from build123d import *

# Parameters (mm, degrees)
F0_W     = 114.3
F0_H     = 127
F0_R     = 38.1
F1_DEPTH = 4.7625
F2_SIZE  = 25.4
F3_SIZE  = 1.524
F4_SIZE  = 3.175


with BuildPart() as f1:
    # F0 (on Top) → F1 (new body, symmetric)
    with BuildSketch(Plane.XY):
        Rectangle(F0_W, F0_H)
        Circle(F0_R, mode=Mode.SUBTRACT)
    extrude(amount=F1_DEPTH, both=True)

    # F2
    f2_edges = [f1.edges().sort_by_distance(p)[0] for p in [
        (57.15, 63.5, 0),
        (-57.15, 63.5, 0),
    ]]
    chamfer(f2_edges, length=F2_SIZE)

    # F3
    f3_edges = [f1.edges().sort_by_distance(p)[0] for p in [
        (-38.1, 0, 4.7625),
        (-38.1, 0, -4.7625),
    ]]
    chamfer(f3_edges, length=F3_SIZE)

    # F4
    f4_edges = [f1.edges().sort_by_distance(p)[0] for p in [
        (0, -63.5, 4.7625),
        (0, -63.5, -4.7625),
    ]]
    chamfer(f4_edges, length=F4_SIZE)


solid = f1.part
Input: part model. Units: mm. Frame: model coordinates. Round coordinates to 2 decimals unless told otherwise and drop trailing zeros. Loops run counter-clockwise (first coordinate to the right, second up) from the corner with the lowest first, then second, coordinate; pieces in that order, holes last. Notation, with made-up numbers: M 82.5,-4 L 138.5,-4 A25 cw 138.5,14 Z; hole C 59.5,30 d10. An arc over 180 degrees is marked long. Answer as CSV lines item,"result". Start each with the question number.
(1) Section B-B, the plane x = 0. Output: boundary loops of the cut face in (y, z) (1 decimal), plus the area to 3 significant figures.
(2) Draft query along Y for faces 1 (the flat face through (-0.8, -61.935, -3.153)), 2 (the flat face through (44.27, 50.98, 0.07)), 3 (the flat face through (-57.15, -13, 0)), 4 (the cylindrical face through (-30.235, -23.183, -0.045)). Return one class per face: released by +Y, released by -Y, zero draft, split by the parting line, or undercut.
(3) Section D-D, the plane y = 43. Output: boundary loops of the cut face in (x, z), plus the area to 3 significant figures.
(4) First-contact query: pin 1 (1 mm diameter, centred on x = 19.5, y = -30, fed in from -Z); pin 2 (2 mm diameter, centred on x = 39.5, z = -3, fed in from -Y); pin 3 (1 mm diameter, centred on x = -37.5, z = 0.5, fed in from +Y). Flat tips, straight axial feed; report the tip coordinate or a pass-through.
(5) Line query: line 1 (Y direction, x = 0, z = 0.5); line 2 (X direction, y = -17.5, z = -0.5); line 3 (Y direction, x = -31, z = -1.25). Output: solid intervals per line, ascending. Write a range as [from, to].
(6) Section A-A, the plane y = 0. Output: boundary loops of the cut face in (x, z), plus the area to 3 significant figures.
Values found:
1,outline,"M -63.5,-1.6 L -60.3,-4.8 L -39.6,-4.8 L -38.1,-3.2 L -38.1,3.2 L -39.6,4.8 L -60.3,4.8 L -63.5,1.6 Z; M 38.1,-3.2 L 39.6,-4.8 L 63.5,-4.8 L 63.5,4.8 L 39.6,4.8 L 38.1,3.2 Z"
1,area,"469 mm²"
2,face 1,"released by -Y"
2,face 2,"released by +Y"
2,face 3,"zero draft"
2,face 4,"undercut"
3,outline,"M -52.25,-4.76 L 52.25,-4.76 L 52.25,4.76 L -52.25,4.76 Z"
3,area,"995 mm²"
4,pin 1,"passes through"
4,pin 2,"stops at y = -63.09"
4,pin 3,"stops at y = 58.25"
5,line 1,"y = [-63.5, -38.1], [38.1, 63.5]"
5,line 2,"x = [-57.15, -33.84], [33.84, 57.15]"
5,line 3,"y = [-63.5, -22.15], [22.15, 63.5]"
6,outline,"M -57.15,-4.76 L -39.62,-4.76 L -38.1,-3.24 L -38.1,3.24 L -39.62,4.76 L -57.15,4.76 Z; M 38.1,-3.24 L 39.62,-4.76 L 57.15,-4.76 L 57.15,4.76 L 39.62,4.76 L 38.1,3.24 Z"
6,area,"358 mm²"
